```python
from build123d import *

# Parameters (mm, degrees)
F0_R     = 63.5
F1_DEPTH = 127
F1_TAPER = -20
F2_SIZE  = 50.8
F3_R     = 25.4
F4_T     = -2.54


# Not quite as in the source:
# - a shell that OpenCascade refuses in one call is made with other operations: the cavity is built on its own and cut out


with BuildPart() as f1:
    # F0 (on Front) → F1 (new body, symmetric)
    with BuildSketch(Plane.XZ):
        Circle(F0_R)
    extrude(amount=F1_DEPTH, both=True, taper=F1_TAPER)

    # F2
    f2_edges = [f1.edges().sort_by_distance(p)[0] for p in [
        (-109.72422, 127, 0),
    ]]
    chamfer(f2_edges, length=F2_SIZE)

    # F3
    f3_edges = [f1.edges().sort_by_distance(p)[0] for p in [
        (-109.72422, -127, 0),
    ]]
    fillet(f3_edges, radius=F3_R)

    # F4: a shell. OpenCascade refuses it in one call, so the cavity is built on its own and cut out:
    # the body offset inwards by the wall thickness, plus a prism from it out through each open face.
    f4_core = offset(f1.part, amount=F4_T, kind=Kind.INTERSECTION, mode=Mode.PRIVATE)
    f4_exits = [f4_core.faces().sort_by_distance(p)[0] for p in [
        (0, -124.46, 0),
    ]]
    add(f4_core, mode=Mode.SUBTRACT)
    extrude(f4_exits, amount=-F4_T, mode=Mode.SUBTRACT)


solid = f1.part
```
CAD build for the part. Positions are in the model's coordinates, mm. A direction names the side the tool comes from. Round coordinates to 2 decimals unless told otherwise and drop trailing zeros. Order: outer loops, then holes, each group sorted by start corner. A loop starts at its lowest first (then second) coordinate and runs counter-clockwise, first axis right, second up.
Q1. Slice it at A-A (x = 81). State how many separate pieces and enclosed holes the cut face has, and give its area (3 significant figures).
Q2. Slice it at D-D (x = 0). Write the cut outline in (y, z).
Q3. Slice it at C-C (y = -63.5). Write the cut outline in (x, z).
Q4. Two-plate mould, pull along Y, no slides. Class faces 1 (the cylindrical face through (70.06, -125.71, -22.06)), 2 (the flat face through (-1, 124.46, 1)), 3 (the conical face through (-14.26, 13.7, -64.22)), 4 (the conical face through (57.75, 124.68, 18.19)): pulls with the +Y half, pulls with the -Y half, needs draft (parallel to the pull), parting line crosses it, or undercut.
Q5. Drop flat-ended pins along their axis: pin 1 (12 mm diameter, centred on y = 96.5, z = -66, fed in from -X); pin 2 (10 mm diameter, centred on x = -63, y = 10, fed in from +Z); pin 3 (8 mm diameter, centred on x = 37.5, z = 68, fed in from -Y). Give the stop position or say it passes through.
Q6. Which spindle directions (+Z, -Z, +X, -X, +Y, -Y) get a long thin tool onto all of the face, cutting with end or side? Do faces 5 (the flat face through (-1, 127, 1)), 6 (the conical face through (-46.94, 122.25, -35.99)). Say none if no direction does.
Q7. Wall check: L1, parallel to Y at x = 40.5, z = -72; L2, parallel to Y at x = -74, z = 53; L3, parallel to Z at x = 7, y = -23. Give the ranges that are in metal, low to high.
Results below:
1. separate pieces: 2
1. enclosed holes: 2
1. area: 2,240 mm2
2. outline: (-127, -73.45) arc R25.4 ccw to (-92.91, -97.32) - (0, -63.5) - (79.26, -92.35) - (127, -58.92) - (127, 58.92) - (79.26, 92.35) - (0, 63.5) - (-92.91, 97.32) arc R25.4 ccw to (-127, 73.45) - (-124.46, 73.45) arc R22.86 cw to (-93.78, 94.93) - (0, 60.8) - (78.89, 89.51) - (124.46, 57.6) - (124.46, -57.6) - (78.89, -89.51) - (0, -60.8) - (-93.78, -94.93) arc R22.86 cw to (-124.46, -73.45) - close
3. outline: circle Ø173.22 at (0, 0); hole circle Ø167.82 at (0, 0)
4. face 1: needs draft
4. face 2: pulls with the -Y half
4. face 3: undercut
4. face 4: pulls with the +Y half
5. pin 1: stops at x = -55.83
5. pin 2: stops at z = 34.55
5. pin 3: stops at y = -127
6. face 5: +Z, -Z, +X, -X, +Y
6. face 6: none
7. L1: y = -125.29 to -122.54, -59.93 to -52.5, 52.5 to 59.93, 88.75 to 93.17
7. L2: y = -119.94 to -116.22, -83.04 to -75.62, 75.62 to 81.16
7. L3: z = -71.53 to -68.81, 68.81 to 71.53
